```python
from build123d import *

# Parameters (mm, degrees)
EXTRUDE_1_DEPTH     = 32
SKETCH_2_R          = 1.5
EXTRUDE_2_DEPTH     = 6
SKETCH_3_R          = 1
CUT_EXTRUDE_1_DEPTH = 10


with BuildPart() as part:
    # 草图1 → 凸台-拉伸1 (new body)
    with BuildSketch(Plane(origin=(0, 0, 0), x_dir=(1, 0, 0), z_dir=(0, 1, 0))):
        Polygon((2.25, 0), (1.125, 1.948557159), (-1.125, 1.948557159), (-2.25, 0), (-1.125, -1.948557159), (1.125, -1.948557159), align=None)
    extrude(amount=EXTRUDE_1_DEPTH)

    # 草图2 → 凸台-拉伸2 (add)
    with BuildSketch(Plane.XZ):
        with Locations(Location((0, 0, 0), (0, 0, 270))):
            Circle(SKETCH_2_R)
    extrude(amount=EXTRUDE_2_DEPTH)

    # 草图3 → 切除-拉伸1 (cut)
    with BuildSketch(Plane(origin=(0, 32, 0), x_dir=(1, 0, 0), z_dir=(0, 1, 0))):
        with Locations(Location((0, 0, 0), (0, 0, 270))):
            Circle(SKETCH_3_R)
    extrude(amount=-CUT_EXTRUDE_1_DEPTH, mode=Mode.SUBTRACT)


solid = part.part
```
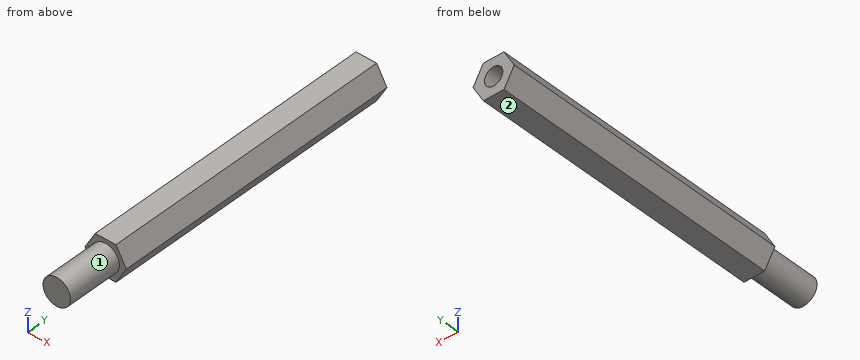
Work out the finished part from the listing and answer in its coordinate system (mm). Face numbers are marked on the shaded views. A direction names the side the tool comes from. Give positions to 0.01 mm unless a question says otherwise; leave off trailing zeros. Write each loop counter-clockwise with the first axis right and the second up, starting at its lowest first coordinate (ties: lowest second). Pieces come first, ordered by that corner, then holes. Notation, with made-up numbers: (-24.5, 79) -> (10.5, 79) arc R14 cw to (10.5, 94) -> close; hole circle Ø9 at (2.25, 10.5). An arc over 180 degrees is marked (long way). Write item = value, one per line.
Q1. Consider line 1 along Z through (x, y) = (-0.8, 26); line 2 along Y through (x, z) = (1.55, -0.5); line 3 along Z through (x, y) = (0.65, 26). Determine where each line is inside the solid, lowest interval first.
Computed values:
line_1 = -1.95 to -0.6, 0.6 to 1.95
line_2 = 0 to 32
line_3 = -1.95 to -0.76, 0.76 to 1.95
Q2. Section A-A on y = 4 is taken. Determine the outline of the cut face in (x, z) (3 decimals).
Computed values:
outline = (-2.25, 0) -> (-1.125, -1.949) -> (1.125, -1.949) -> (2.25, 0) -> (1.125, 1.949) -> (-1.125, 1.949) -> close
Q3. Section B-B on x = 0 is taken. Determine the outline of the cut face in (y, z), and give its area (3 significant figures).
Computed values:
outline = (-6, -1.5) -> (0, -1.5) -> (0, -1.95) -> (32, -1.95) -> (32, -1) -> (22, -1) -> (22, 1) -> (32, 1) -> (32, 1.95) -> (0, 1.95) -> (0, 1.5) -> (-6, 1.5) -> close
area = 123 mm^2
Q4. Flat-ended cylindrical pins translate along their axes: pin 1 Ø1.5 at (y, z) = (5, -1.5) entering from -X; pin 2 Ø1 at (y, z) = (24, -1) entering from -X; pin 3 Ø1.2 at (x, z) = (0, 0) entering from +Y. Find the tip coordinate at first contact, or state that the pin passes through.
Computed values:
pin_1 = -1.82
pin_2 = -1.96
pin_3 = 22
Q5. Section C-C on z = -0.6 is taken. Determine the outline of the cut face in (x, y).
Computed values:
outline = (-1.9, 0) -> (-1.37, 0) -> (-1.37, -6) -> (1.37, -6) -> (1.37, 0) -> (1.9, 0) -> (1.9, 32) -> (0.8, 32) -> (0.8, 22) -> (-0.8, 22) -> (-0.8, 32) -> (-1.9, 32) -> close
Q6. A tool of negligible diameter and unlimited length cuts with its end or side. For the marked faces 1 and 2, from which of +Z, -Z, +X, -X, +Y, -Y can it reach the whole face along a straight path? Write none if from no direction.
Computed values:
face_1 = -Y
face_2 = -Z, +X, -X, +Y, -Y
